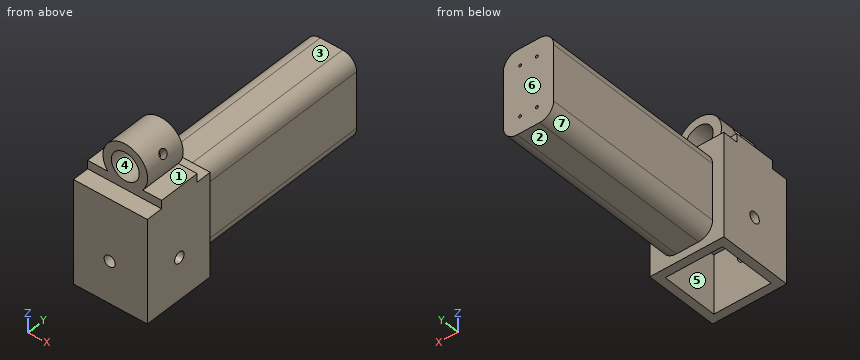
from build123d import *

# Parameters (mm, degrees)
ESQUISSE1_W                   = 26.5
ESQUISSE1_H                   = 26.5
BOSS_EXTRU_1_DEPTH            = 40
ESQUISSE2_W                   = 20.5
ESQUISSE2_H                   = 20.5
ENL_V_MAT_EXTRU_1_DEPTH       = 21
ESQUISSE4_R                   = 8
ESQUISSE4_R_2                 = 5
BOSS_EXTRU_3_DEPTH            = 7.5
ESQUISSE4_4_R                 = 8
ESQUISSE4_4_R_2               = 5
BOSS_EXTRU_4_DEPTH            = 7.5
ESQUISSE8_W                   = 26.5
ESQUISSE8_H                   = 3
ENL_V_MAT_EXTRU_4_DEPTH       = 6
ESQUISSE12_W                  = 18
ESQUISSE12_H                  = 30
BOSS_EXTRU_5_DEPTH            = 67
CONG_1_R                      = 5
CONG_2_R                      = 5
CONG_3_R                      = 5
CONG_4_R                      = 5
ENL_V_MAT_EXTRU_7_REACH       = 51.366
ESQUISSE17_R                  = 1.5
ENL_V_MAT_EXTRU_8_REACH       = 51.012
ESQUISSE18_R                  = 1.5
ESQUISSE13_R                  = 0.5
ENL_V_MAT_EXTRU_9_DEPTH       = 5
ESQUISSE19_R                  = 2
ENL_V_MAT_EXTRU_10_DEPTH      = 1
ENL_V_MAT_EXTRU_10_DEPTH_BACK = 27.5
ENL_V_MAT_EXTRU_11_REACH      = 95.5
ESQUISSE20_R                  = 2
ESQUISSE9_W                   = 26.5
ESQUISSE9_H                   = 3
ENL_V_MAT_EXTRU_13_DEPTH      = 5.5


with BuildPart() as part:
    # Esquisse1 → Boss.-Extru.1 (new body)
    with BuildSketch(Plane.XY):
        with Locations((0.553632827, -1.655537459)):
            Rectangle(ESQUISSE1_W, ESQUISSE1_H)
    extrude(amount=BOSS_EXTRU_1_DEPTH)

    # Esquisse2 → Enlèv. mat.-Extru.1 (cut)
    with BuildSketch(Plane(origin=(0, 0, 0), x_dir=(-1, 0, 0), z_dir=(0, 0, -1))):
        with Locations((-0.553632827, -1.655537459)):
            Rectangle(ESQUISSE2_W, ESQUISSE2_H)
    extrude(amount=-ENL_V_MAT_EXTRU_1_DEPTH, mode=Mode.SUBTRACT)

    # Esquisse4 → Boss.-Extru.3 (add)
    with BuildSketch(Plane(origin=(0, -1.405537459, 0), x_dir=(-1, 0, 0), z_dir=(0, -1, 0))):
        with Locations((-0.803632827, -45)):
            Circle(ESQUISSE4_R)
        with Locations((-0.803632827, -45)):
            Circle(ESQUISSE4_R_2, mode=Mode.SUBTRACT)
    extrude(amount=BOSS_EXTRU_3_DEPTH)

    # Esquisse4<4> → Boss.-Extru.4 (add)
    with BuildSketch(Plane(origin=(0, -1.405537459, 0), x_dir=(-1, 0, 0), z_dir=(0, -1, 0))):
        with Locations((-0.803632827, -45)):
            Circle(ESQUISSE4_4_R)
        with Locations((-0.803632827, -45)):
            Circle(ESQUISSE4_4_R_2, mode=Mode.SUBTRACT)
    extrude(amount=-BOSS_EXTRU_4_DEPTH)

    # Esquisse8 → Enlèv. mat.-Extru.4 (cut)
    with BuildSketch(Plane.XZ.offset(14.905537459)):
        with Locations((0.553632827, 38.5)):
            Rectangle(ESQUISSE8_W, ESQUISSE8_H)
    extrude(amount=-ENL_V_MAT_EXTRU_4_DEPTH, mode=Mode.SUBTRACT)

    # Esquisse12 → Boss.-Extru.5 (add)
    with BuildSketch(Plane(origin=(0, 11.594462541, 0), x_dir=(1, 0, 0), z_dir=(0, 1, 0))):
        with Locations((0.303632827, -18)):
            Rectangle(ESQUISSE12_W, ESQUISSE12_H)
    extrude(amount=BOSS_EXTRU_5_DEPTH)

    # Congé1
    cong_1_edges = [part.edges().sort_by_distance(p)[0] for p in [
        (9.303632827, 45.094462541, 33),
    ]]
    fillet(cong_1_edges, radius=CONG_1_R)

    # Congé2
    cong_2_edges = [part.edges().sort_by_distance(p)[0] for p in [
        (-8.696367173, 45.094462541, 33),
    ]]
    fillet(cong_2_edges, radius=CONG_2_R)

    # Congé3
    cong_3_edges = [part.edges().sort_by_distance(p)[0] for p in [
        (-8.696367173, 45.094462541, 3),
    ]]
    fillet(cong_3_edges, radius=CONG_3_R)

    # Congé4
    cong_4_edges = [part.edges().sort_by_distance(p)[0] for p in [
        (9.303632827, 45.094462541, 3),
    ]]
    fillet(cong_4_edges, radius=CONG_4_R)

    # Esquisse17 → Enlèv. mat.-Extru.7 (cut, up to next)
    with BuildSketch(Plane(origin=(28.558670663, 0, 28.558670663), x_dir=(0.707106781, 0, -0.707106781), z_dir=(0.707106781, 0, 0.707106781)), mode=Mode.PRIVATE) as enl_v_mat_extru_7_sk1:
        with Locations((-28.738974236, -1.405537459)):
            Circle(ESQUISSE17_R)
    enl_v_mat_extru_7_tool1 = extrude(enl_v_mat_extru_7_sk1.sketch, amount=-ENL_V_MAT_EXTRU_7_REACH, mode=Mode.PRIVATE) & part.part
    add(enl_v_mat_extru_7_tool1.solids().sort_by_distance((8.237147, -1.405537, 48.880194))[0], mode=Mode.SUBTRACT)

    # Esquisse18 → Enlèv. mat.-Extru.8 (cut, up to next)
    with BuildSketch(Plane(origin=(-27.755037836, 0, 27.755037836), x_dir=(0.707106781, 0, 0.707106781), z_dir=(-0.707106781, 0, 0.707106781)), mode=Mode.PRIVATE) as enl_v_mat_extru_8_sk1:
        with Locations((29.875394998, -1.405537459)):
            Circle(ESQUISSE18_R)
    enl_v_mat_extru_8_tool1 = extrude(enl_v_mat_extru_8_sk1.sketch, amount=-ENL_V_MAT_EXTRU_8_REACH, mode=Mode.PRIVATE) & part.part
    add(enl_v_mat_extru_8_tool1.solids().sort_by_distance((-6.629943, -1.405537, 48.880132))[0], mode=Mode.SUBTRACT)

    # Esquisse13 → Enlèv. mat.-Extru.9 (cut)
    with BuildSketch(Plane(origin=(0, 78.594462541, 0), x_dir=(1, 0, 0), z_dir=(0, 1, 0))):
        with Locations((3.303632827, -9)):
            Circle(ESQUISSE13_R)
        with Locations((-2.696367173, -9)):
            Circle(ESQUISSE13_R)
        with Locations((3.303632827, -27)):
            Circle(ESQUISSE13_R)
        with Locations((-2.696367173, -27)):
            Circle(ESQUISSE13_R)
    extrude(amount=-ENL_V_MAT_EXTRU_9_DEPTH, mode=Mode.SUBTRACT)

    # Esquisse19 → Enlèv. mat.-Extru.10 (cut, two sides)
    with BuildSketch(Plane.ZY.offset(12.696367173)) as enl_v_mat_extru_10_sk:
        with Locations((15, -1.405537459)):
            Circle(ESQUISSE19_R)
    extrude(amount=ENL_V_MAT_EXTRU_10_DEPTH, mode=Mode.SUBTRACT)
    extrude(enl_v_mat_extru_10_sk.sketch, amount=-ENL_V_MAT_EXTRU_10_DEPTH_BACK, mode=Mode.SUBTRACT)

    # Esquisse20 → Enlèv. mat.-Extru.11 (cut, up to next)
    with BuildSketch(Plane.XZ.offset(14.905537459), mode=Mode.PRIVATE) as enl_v_mat_extru_11_sk1:
        with Locations((0.303632827, 15)):
            Circle(ESQUISSE20_R)
    enl_v_mat_extru_11_tool1 = extrude(enl_v_mat_extru_11_sk1.sketch, amount=-ENL_V_MAT_EXTRU_11_REACH, mode=Mode.PRIVATE) & part.part
    add(enl_v_mat_extru_11_tool1.solids().sort_by_distance((0.303633, -14.905537, 15))[0], mode=Mode.SUBTRACT)

    # Esquisse9 → Enlèv. mat.-Extru.13 (cut)
    with BuildSketch(Plane(origin=(0, 11.594462541, 0), x_dir=(1, 0, 0), z_dir=(0, 1, 0))):
        with Locations((0.553632827, -38.5)):
            Rectangle(ESQUISSE9_W, ESQUISSE9_H)
    extrude(amount=-ENL_V_MAT_EXTRU_13_DEPTH, mode=Mode.SUBTRACT)


solid = part.part
Check sheet for the modelled part. Datum: model origin and axes. Units: mm. Face numbers are marked on the shaded views. A direction names the side the tool comes from. Coordinates: 2 decimals unless noted, no trailing zeros. Write each loop counter-clockwise with the first axis right and the second up, starting at its lowest first coordinate (ties: lowest second). Pieces come first, ordered by that corner, then holes.
Item 1: Access from +Z, -Z, +X, -X, +Y, -Y to the whole of each face (thin tool, end or side, straight path). Record for the marked faces 1, 2 and 3.
Numbers:
face 1: +X, +Y, -Y
face 2: -Z, +X, -X, +Y
face 3: +Z, +X, -X, +Y
Item 2: Cross-section at B-B on y = 62. Record the boundary of the cut face in (x, z).
Numbers:
outline: (-8.7, 8) arc R5 ccw to (-3.7, 3) - (4.3, 3) arc R5 ccw to (9.3, 8) - (9.3, 28) arc R5 ccw to (4.3, 33) - (-3.7, 33) arc R5 ccw to (-8.7, 28) - close
Item 3: Cross-section at A-A on z = 10.5. Record the boundary of the cut face in (x, y), then the cut area to 3 significant figures.
Numbers:
outline: (-12.7, -14.91) - (13.8, -14.91) - (13.8, 11.59) - (9.3, 11.59) - (9.3, 78.59) - (-8.7, 78.59) - (-8.7, 11.59) - (-12.7, 11.59) - close; hole (-9.7, -11.91) - (10.8, -11.91) - (10.8, 8.59) - (-9.7, 8.59) - close
area: 1,490 mm2
Item 4: Mould release check, pull along X, two halves, no side actions. Record for the marked faces 4, 5, 6 and 7: released by +X, released by -X, zero draft, split by the parting line, or undercut.
Numbers:
face 4: undercut
face 5: undercut
face 6: zero draft
face 7: released by -X
Item 5: Cross-section at C-C on x = -11. Record the boundary of the cut face in (y, z), then the cut area to 3 significant figures.
Numbers:
outline: (-14.91, 0) - (11.59, 0) - (11.59, 37) - (6.09, 37) - (6.09, 40) - (-8.91, 40) - (-8.91, 37) - (-14.91, 37) - close; hole circle Ø4 at (-1.41, 15)
area: 1,010 mm2
Item 6: Depth check by flat-ended pin: pin 1 Ø6 at (x, z) = (0.8, 45) entering from +Y (1 decimal); pin 2 Ø9 at (x, y) = (0, 56.5) entering from +Z; pin 3 Ø6 at (y, z) = (51, 17.5) entering from +X; pin 4 Ø6.5 at (x, y) = (-6, -13) entering from +Z. Enter the tip coordinate at first touch or a pass-through.
Numbers:
pin 1: passes through
pin 2: stops at z = 33
pin 3: stops at x = 9.3
pin 4: stops at z = 37
Item 7: Scan lines: probe 1 along X at (y, z) = (75, 27); probe 2 along X at (y, z) = (-9.5, 5); probe 3 along Y at (x, z) = (5, 20.5). Record each from-to range of solid material in increasing order.
Numbers:
probe 1: x = -8.7 to -3.2, -2.2 to 2.8, 3.8 to 9.3
probe 2: x = -12.7 to -9.7, 10.8 to 13.8
probe 3: y = -14.91 to -11.91, 8.59 to 78.59
